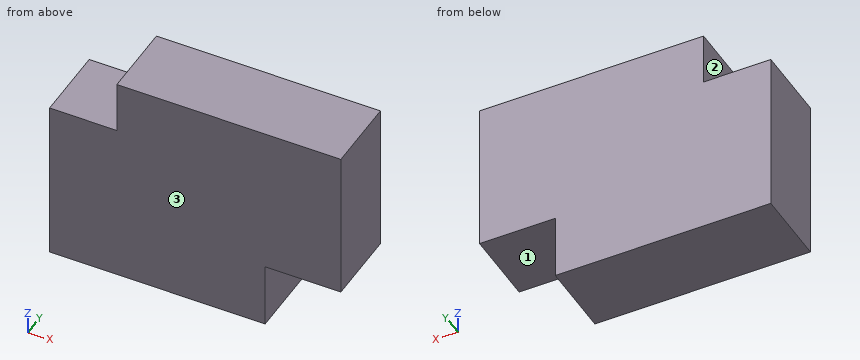
```python
from build123d import *

# Parameters (mm, degrees)
F0_W     = 49.7014243156
F0_H     = 33.4998108447
F1_DEPTH = 25.4


with BuildPart() as f1:
    # F0 (on Front) → F1 (new body)
    with BuildSketch(Plane.XZ):
        Polygon((-45.1190248132, 60.9986558557), (-45.1190248132, 43.2065278292), (4.5823995024, 43.2065278292), (4.5823995024, 9.7067169845), (29.9618467689, 9.7067169845), (29.9618467689, 60.9986558557), align=None)
        Polygon((-45.1190248132, 43.2065278292), (-67.6785334945, 43.2065278292), (-67.6785334945, -12.4243786559), (4.5823995024, -12.4243786559), (4.5823995024, 9.7067169845), (-45.1190248132, 9.7067169845), align=None)
        with Locations((-20.2683126554, 26.4566224068)):
            Rectangle(F0_W, F0_H)
    extrude(amount=F1_DEPTH)


solid = f1.part
```
Read the model definition and answer for the solid it produces. Units are mm, in the model's axes. Face numbers are marked on the shaded views. A direction names the side the tool comes from. Give positions to 0.01 mm unless a question says otherwise; leave off trailing zeros. Write each loop counter-clockwise with the first axis right and the second up, starting at its lowest first coordinate (ties: lowest second). Pieces come first, ordered by that corner, then holes. Notation, with made-up numbers: (85, 74.25) -> (96, 74.25) arc R16 cw to (96, 84.25) -> close; hole circle Ø2 at (-8.5, -10.75). An arc over 180 degrees is marked (long way). Answer as a JSON object with one key per item and string values.
1) Flat-ended cylindrical pins translate along their axes: pin 1 Ø9 at (y, z) = (-16, 54) entering from -X; pin 2 Ø12.5 at (x, y) = (23, -17.5) entering from -Z. Find the tip coordinate at first contact, or state that the pin passes through.
Findings below:
{"pin 1": "stops at x = -45.12", "pin 2": "stops at z = 9.71"}
2) Straight lines are drawn through the part: probe 1 along X at (y, z) = (-17, 0); probe 2 along Z at (x, y) = (9.5, -2.5); probe 3 along X at (y, z) = (-0.75, 46). For each, find the intervals that lie inside material, in ascending order. Write a range as from..to.
Findings below:
{"probe 1": "x = -67.68..4.58", "probe 2": "z = 9.71..61", "probe 3": "x = -45.12..29.96"}
3) Section C-C on x = -54.5 is taken. Write down the section's boundary in (y, z), then the cut area to 3 significant figures.
Findings below:
{"outline": "(-25.4, -12.42) -> (0, -12.42) -> (0, 43.21) -> (-25.4, 43.21) -> close", "area": "1,410 mm^2"}
4) Section B-B on z = 55 is taken. Write down the section's boundary in (x, y), then the cut area to 3 significant figures.
Findings below:
{"outline": "(-45.12, -25.4) -> (29.96, -25.4) -> (29.96, 0) -> (-45.12, 0) -> close", "area": "1,910 mm^2"}
5) Section A-A on y = -3.75 is taken. Write down the section's boundary in (x, z).
Findings below:
{"outline": "(-67.68, -12.42) -> (4.58, -12.42) -> (4.58, 9.71) -> (29.96, 9.71) -> (29.96, 61) -> (-45.12, 61) -> (-45.12, 43.21) -> (-67.68, 43.21) -> close"}
6) A tool of negligible diameter and unlimited length cuts with its end or side. For the marked faces 1, 2 and 3, from which of +Z, -Z, +X, -X, +Y, -Y can it reach the whole face along a straight path? Write none if from no direction.
Findings below:
{"face 1": "-Z, +X, +Y, -Y", "face 2": "+Z, -X, +Y, -Y", "face 3": "+Z, -Z, +X, -X, -Y"}
